For this review, take the finished solid that the model builds, in its own axes (mm). Face numbers are marked on the shaded views. A direction names the side the tool comes from. Give positions to 0.01 mm unless a question says otherwise; leave off trailing zeros. Loops run counter-clockwise (first coordinate to the right, second up) from the corner with the lowest first, then second, coordinate; pieces in that order, holes last. Notation, with made-up numbers: (-21, 46) -> (35, 46) arc R24 cw to (35, 81) -> close; hole circle Ø5 at (50.25, -12). An arc over 180 degrees is marked (long way). One line per question, with ' | ' between items. Start each with the question number.
(1) Consider section A-A (x = -79). Write out the cut boundary in (y, z).
(2) Insertion check: P1, Ø1, axis at x = -68, z = 20.5, coming from the -Y side; P2, Ø6, axis at x = 94, y = -54, coming from the -Z side; P3, Ø12, axis at x = 29.5, y = -77, coming from the +Z side. Each pin has a flat end and moves straight along its axis. Give the tip position at first contact, or say it passes through.
(3) Tool access review of the marked faces 1, 2 and 3: name each direction out of +Z, -Z, +X, -X, +Y, -Y from which nothing blocks a thin tool from reaching the whole face with its end or side.
(4) Wall thickness on probe 1 along Z at (x, y) = (98.5, -43.5); probe 2 along Z at (x, y) = (-95.5, -51); probe 3 along Y at (x, z) = (48, -9): over which ranges is each line inside the solid? List them lowest first.
from build123d import *

# Parameters (mm, degrees)
F0_W     = 250
F0_H     = 60
F1_DEPTH = 60
F3_DEPTH = 250
F8_R     = 5


with BuildPart() as f1:
    # F0 (on Front) → F1 (new body)
    with BuildSketch(Plane.XZ):
        Rectangle(F0_W, F0_H)
    extrude(amount=F1_DEPTH)

    # F2 (on face) → F3 (cut)
    with BuildSketch(Plane.YZ.offset(125)):
        Polygon((-60, -30), (0, 30), (-60, 30), align=None)
    extrude(amount=-F3_DEPTH, mode=Mode.SUBTRACT)

    # F4 (on face) → F7 section 0
    with BuildSketch(Plane(origin=(0, 0, 0), x_dir=(-1, 0, 0), z_dir=(0, 1, 0))):
        Polygon((35, 30), (-35, 30), (-30, -30), (30, -30), align=None)
    # F6 (on offset) → F7 section 1
    with BuildSketch(Plane.XZ.offset(95)):
        Polygon((25, 14.1158560291), (-25, 14.1158560291), (-29.863614589, -30.5979736149), (30.136385411, -30.5979736149), align=None)
    loft()

    # F8
    f8_edges = [f1.edges().sort_by_distance(p)[0] for p in [
        (30, -47.5, 22.057928),
        (-30, -47.5, 22.057928),
    ]]
    fillet(f8_edges, radius=F8_R)


solid = f1.part
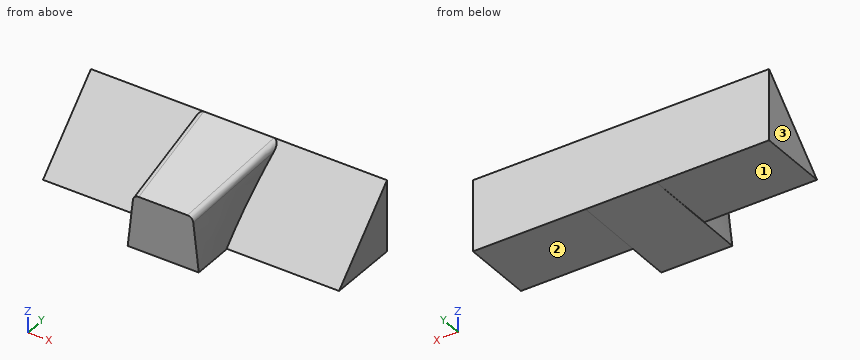
A:
1) outline: (-60, -30) -> (0, -30) -> (0, 30) -> close
2) P1: stops at y = -10 | P2: stops at z = -30 | P3: stops at z = 17.31
3) face 1: -Z, -X, +Y, -Y | face 2: -Z, +X, +Y, -Y | face 3: +Z, -Z, -X, +Y, -Y
4) probe 1: z = -30 to -13.5 | probe 2: z = -30 to -21 | probe 3: y = -39 to 0
